Autodesk Inventor part; units mm, degrees
ref_plane "YZ Plane" through (0, 0, 0) normal (1, 0, 0) x (0, 1, 0)
ref_plane "XZ Plane" through (0, 0, 0) normal (0, 1, 0) x (-1, 0, 0)
ref_plane "XY Plane" through (0, 0, 0) normal (0, 0, 1) x (1, 0, 0)
sketch "Sketch1" plane through (0, 0, 0) normal (1, 0, 0) x (0, 1, 0)
  line L0 (0, 0) -> (-25.4, 0)
  line L1 (-25.4, 0) -> (-25.4, -25.4)
  line L2 (-25.4, -25.4) -> (0, -25.4)
  line L3 (0, -25.4) -> (0, 0)
  line L4 (-1.5875, -23.8125) -> (-23.8125, -23.8125)
  line L5 (-23.8125, -23.8125) -> (-23.8125, -1.5875)
  line L6 (-23.8125, -1.5875) -> (-1.5875, -1.5875)
  line L7 (-1.5875, -1.5875) -> (-1.5875, -23.8125)
  point P0 (-12.7, -23.8125)
  point P1 (-12.7, -25.4)
  point P2 (-23.8125, -12.7)
  point P3 (-1.5875, -12.7)
  dimension "d0" = 25.4
  dimension "d1" = 25.4
  dimension "d2" = 1.5875
  dimension "d3" = 1.5875
  dimension "d4" = 1.5875
  dimension "d5" = 1.5875
extrude "Extrusion1" add sketch "Sketch1" along normal blind 558.8
properties part number "44.92cmTube" material "Aluminum 6061"
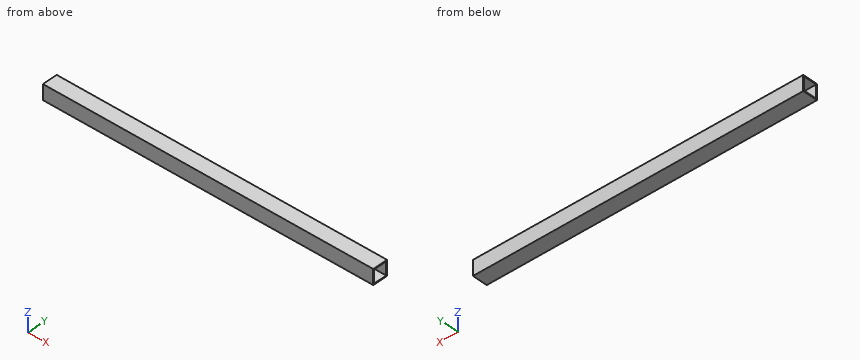
For this review, take the finished solid that the model builds, in its own axes (mm). Round coordinates to 2 decimals unless told otherwise and drop trailing zeros. Write each loop counter-clockwise with the first axis right and the second up, starting at its lowest first coordinate (ties: lowest second). Pieces come first, ordered by that corner, then holes. Notation, with made-up numbers: M 81,24 L 136,24 A21 cw 136,43 Z; hole C -11,74.25 d1. An arc over 180 degrees is marked long. One line per item, written item: value. Start each with the question number.
(1) We need section C-C (x = 109.5). Give the boundary of the cut face in (y, z).
(2) Wall thickness on line 1 (Z direction, x = 436, y = -16): over which ranges is the line inside the solid? List them lowest first.
(3) We need section A-A (z = -14.25). Give the boundary of the cut face in (x, y), and give its area (3 significant figures).
Result:
1. outline: M -25.4,-25.4 L 0,-25.4 L 0,0 L -25.4,0 Z; hole M -23.81,-23.81 L -1.59,-23.81 L -1.59,-1.59 L -23.81,-1.59 Z
2. line 1: -25.4 to -23.81, -1.59 to 0
3. outline: M 0,-25.4 L 558.8,-25.4 L 558.8,-23.81 L 0,-23.81 Z; M 0,-1.59 L 558.8,-1.59 L 558.8,0 L 0,0 Z
3. area: 1,770 mm²
